```python
from build123d import *

# Parameters (mm, degrees)
SKETCH058_W     = 445
SKETCH058_H     = 232
PAD022_DEPTH    = 3
SKETCH059_R     = 9.5
POCKET036_DEPTH = 5
FILLET007_R     = 2
SKETCH060_R     = 7
POCKET037_DEPTH = 10.001
SKETCH079_W     = 462.91922
SKETCH079_H     = 530.257522
POCKET051_DEPTH = 5


with BuildPart() as part:
    # Sketch058 → Pad022 (new body)
    with BuildSketch(Plane.XY):
        Rectangle(SKETCH058_W, SKETCH058_H)
    extrude(amount=PAD022_DEPTH)

    # Sketch059 (on Face6 of Pad022) → Pocket036 (cut)
    with BuildSketch(Plane.XY.offset(3)):
        with Locations((-171, 55)):
            Circle(SKETCH059_R)
        with Locations((-171, 33)):
            Circle(SKETCH059_R)
        with Locations((-171, 11)):
            Circle(SKETCH059_R)
        with Locations((-171, -11)):
            Circle(SKETCH059_R)
        with Locations((-171, -33)):
            Circle(SKETCH059_R)
        with Locations((-171, -55)):
            Circle(SKETCH059_R)
        with Locations((-152, 44)):
            Circle(SKETCH059_R)
        with Locations((-152, 22)):
            Circle(SKETCH059_R)
        with Locations((-152, 0)):
            Circle(SKETCH059_R)
        with Locations((-152, -22)):
            Circle(SKETCH059_R)
        with Locations((-152, -44)):
            Circle(SKETCH059_R)
        with Locations((-133, 55)):
            Circle(SKETCH059_R)
        with Locations((-133, 33)):
            Circle(SKETCH059_R)
        with Locations((-133, 11)):
            Circle(SKETCH059_R)
        with Locations((-133, -11)):
            Circle(SKETCH059_R)
        with Locations((-133, -33)):
            Circle(SKETCH059_R)
        with Locations((-133, -55)):
            Circle(SKETCH059_R)
        with Locations((-114, 44)):
            Circle(SKETCH059_R)
        with Locations((-114, 22)):
            Circle(SKETCH059_R)
        with Locations((-114, 0)):
            Circle(SKETCH059_R)
        with Locations((-114, -22)):
            Circle(SKETCH059_R)
        with Locations((-114, -44)):
            Circle(SKETCH059_R)
        with Locations((-95, 55)):
            Circle(SKETCH059_R)
        with Locations((-95, 33)):
            Circle(SKETCH059_R)
        with Locations((-95, 11)):
            Circle(SKETCH059_R)
        with Locations((-95, -11)):
            Circle(SKETCH059_R)
        with Locations((-95, -33)):
            Circle(SKETCH059_R)
        with Locations((-95, -55)):
            Circle(SKETCH059_R)
        with Locations((-76, -44)):
            Circle(SKETCH059_R)
        with Locations((-76, -22)):
            Circle(SKETCH059_R)
        with Locations((-76, 0)):
            Circle(SKETCH059_R)
        with Locations((-76, 22)):
            Circle(SKETCH059_R)
        with Locations((-76, 44)):
            Circle(SKETCH059_R)
        with Locations((-57, 55)):
            Circle(SKETCH059_R)
        with Locations((-57, 33)):
            Circle(SKETCH059_R)
        with Locations((-57, 11)):
            Circle(SKETCH059_R)
        with Locations((-57, -11)):
            Circle(SKETCH059_R)
        with Locations((-57, -33)):
            Circle(SKETCH059_R)
        with Locations((-38, 44)):
            Circle(SKETCH059_R)
        with Locations((-38, 22)):
            Circle(SKETCH059_R)
        with Locations((-38, 0)):
            Circle(SKETCH059_R)
        with Locations((-38, -22)):
            Circle(SKETCH059_R)
        with Locations((-38, -44)):
            Circle(SKETCH059_R)
        with Locations((-57, -55)):
            Circle(SKETCH059_R)
        with Locations((-19, 55)):
            Circle(SKETCH059_R)
        with Locations((-19, 33)):
            Circle(SKETCH059_R)
        with Locations((-19, 11)):
            Circle(SKETCH059_R)
        with Locations((-19, -11)):
            Circle(SKETCH059_R)
        with Locations((-19, -33)):
            Circle(SKETCH059_R)
        with Locations((-19, -55)):
            Circle(SKETCH059_R)
        with Locations((0, -44)):
            Circle(SKETCH059_R)
        with Locations((0, -22)):
            Circle(SKETCH059_R)
        Circle(SKETCH059_R)
        with Locations((0, 22)):
            Circle(SKETCH059_R)
        with Locations((0, 44)):
            Circle(SKETCH059_R)
        with Locations((19, 55)):
            Circle(SKETCH059_R)
        with Locations((19, 33)):
            Circle(SKETCH059_R)
        with Locations((19, 11)):
            Circle(SKETCH059_R)
        with Locations((19, -11)):
            Circle(SKETCH059_R)
        with Locations((19, -33)):
            Circle(SKETCH059_R)
        with Locations((19, -55)):
            Circle(SKETCH059_R)
        with Locations((38, -44)):
            Circle(SKETCH059_R)
        with Locations((38, -22)):
            Circle(SKETCH059_R)
        with Locations((38, 0)):
            Circle(SKETCH059_R)
        with Locations((38, 22)):
            Circle(SKETCH059_R)
        with Locations((38, 44)):
            Circle(SKETCH059_R)
        with Locations((57, 55)):
            Circle(SKETCH059_R)
        with Locations((57, 33)):
            Circle(SKETCH059_R)
        with Locations((57, 11)):
            Circle(SKETCH059_R)
        with Locations((57, -11)):
            Circle(SKETCH059_R)
        with Locations((76, 0)):
            Circle(SKETCH059_R)
        with Locations((76, 22)):
            Circle(SKETCH059_R)
        with Locations((76, 44)):
            Circle(SKETCH059_R)
        with Locations((57, -33)):
            Circle(SKETCH059_R)
        with Locations((57, -55)):
            Circle(SKETCH059_R)
        with Locations((76, -44)):
            Circle(SKETCH059_R)
        with Locations((76, -22)):
            Circle(SKETCH059_R)
        with Locations((95, 55)):
            Circle(SKETCH059_R)
        with Locations((95, 33)):
            Circle(SKETCH059_R)
        with Locations((95, 11)):
            Circle(SKETCH059_R)
        with Locations((95, -11)):
            Circle(SKETCH059_R)
        with Locations((95, -33)):
            Circle(SKETCH059_R)
        with Locations((95, -55)):
            Circle(SKETCH059_R)
        with Locations((114, 44)):
            Circle(SKETCH059_R)
        with Locations((114, 22)):
            Circle(SKETCH059_R)
        with Locations((114, 0)):
            Circle(SKETCH059_R)
        with Locations((114, -22)):
            Circle(SKETCH059_R)
        with Locations((114, -44)):
            Circle(SKETCH059_R)
        with Locations((133, 55)):
            Circle(SKETCH059_R)
        with Locations((133, 33)):
            Circle(SKETCH059_R)
        with Locations((133, 11)):
            Circle(SKETCH059_R)
        with Locations((133, -11)):
            Circle(SKETCH059_R)
        with Locations((133, -33)):
            Circle(SKETCH059_R)
        with Locations((133, -55)):
            Circle(SKETCH059_R)
        with Locations((152, 44)):
            Circle(SKETCH059_R)
        with Locations((152, 22)):
            Circle(SKETCH059_R)
        with Locations((152, 0)):
            Circle(SKETCH059_R)
        with Locations((152, -22)):
            Circle(SKETCH059_R)
        with Locations((152, -44)):
            Circle(SKETCH059_R)
        with Locations((171, 55)):
            Circle(SKETCH059_R)
        with Locations((171, 33)):
            Circle(SKETCH059_R)
        with Locations((171, 11)):
            Circle(SKETCH059_R)
        with Locations((171, -11)):
            Circle(SKETCH059_R)
        with Locations((171, -33)):
            Circle(SKETCH059_R)
        with Locations((171, -55)):
            Circle(SKETCH059_R)
    extrude(amount=-POCKET036_DEPTH, mode=Mode.SUBTRACT)

    # Fillet007
    fillet007_edges = [part.edges().sort_by_distance(p)[0] for p in [
        (-222.5, -116, 1.5),
        (222.5, -116, 1.5),
        (222.5, 116, 1.5),
        (-222.5, 116, 1.5),
    ]]
    fillet(fillet007_edges, radius=FILLET007_R)

    # Sketch060 → Pocket037 (cut, through all)
    with BuildSketch(Plane.XY.offset(10)):
        with Locations((197.939534, 0)):
            Circle(SKETCH060_R)
    extrude(amount=-POCKET037_DEPTH, mode=Mode.SUBTRACT)

    # Sketch079 (on Face5 of Pocket037) → Pocket051 (cut)
    with BuildSketch(Plane.XY.offset(3)):
        with Locations((-171.45961, -16.154991)):
            Rectangle(SKETCH079_W, SKETCH079_H)
    extrude(amount=-POCKET051_DEPTH, mode=Mode.SUBTRACT)


solid = part.part
```
Verification items for the finished model (mm, model axes). Give positions to 0.01 mm unless a question says otherwise; leave off trailing zeros. Order: outer loops, then holes, each group sorted by start corner. A loop starts at its lowest first (then second) coordinate and runs counter-clockwise, first axis right, second up. Notation, with made-up numbers: M 10,33 L 19,33 A8 ccw 19,37 Z; hole C -33,52.5 d6. An arc over 180 degrees is marked long. Answer in a Markdown table with one row per item. Add a question column.
Item 1: Mould release check, pull along Y, two halves, no side actions. Record for faces 1 (the cylindrical face through (123.51, -10.58, 1.52)), 2 (the flat face through (140, 2, 0)): released by +Y, released by -Y, zero draft, split by the parting line, or undercut.
Item 2: Section check C-C, the plane y = -28. Enter the section's corners in (x, z).
Item 3: Gauge pin test, flat end, axial feed: pin 1 (11.5 mm diameter, centred on x = 95, y = 33, fed in from -Z). Record the tip position at first contact, or that the pin passes through.
Item 4: Section check D-D, the plane z = 1.3. State how many separate pieces and enclosed holes the cut face has, and give its area (3 significant figures).
Item 5: Section check A-A, the plane x = 152. Enter the section's corners in (y, z), and give its area (3 significant figures).
Item 6: Section check B-B, the plane x = 174. Enter the section's corners in (y, z), and give its area (4 significant figures).
Item 7: Scan lines: probe 1 along Y at (x, z) = (76, 0.8); probe 2 along X at (y, z) = (-57.5, 2.7); probe 3 along Y at (x, z) = (72, 1.5). Record each from-to range of solid material in increasing order. Write a range as from..to.
Filled sheet:
| question | item | result |
|---|---|---|
| 1 | face 1 | undercut |
| 1 | face 2 | zero draft |
| 2 | outline | M 65.08,0 L 68.63,0 L 68.63,3 L 65.08,3 Z; M 83.37,0 L 86.92,0 L 86.92,3 L 83.37,3 Z; M 103.08,0 L 106.63,0 L 106.63,3 L 103.08,3 Z; M 121.37,0 L 124.92,0 L 124.92,3 L 121.37,3 Z; M 141.08,0 L 144.63,0 L 144.63,3 L 141.08,3 Z; M 159.37,0 L 162.92,0 L 162.92,3 L 159.37,3 Z; M 179.08,0 L 222.5,0 L 222.5,3 L 179.08,3 Z |
| 3 | pin 1 | passes through |
| 4 | separate pieces | 1 |
| 4 | enclosed holes | 34 |
| 4 | area | 27,700 mm^2 |
| 5 | outline | M -116,0 L -53.5,0 L -53.5,3 L -116,3 Z; M -34.5,0 L -31.5,0 L -31.5,3 L -34.5,3 Z; M -12.5,0 L -9.5,0 L -9.5,3 L -12.5,3 Z; M 9.5,0 L 12.5,0 L 12.5,3 L 9.5,3 Z; M 31.5,0 L 34.5,0 L 34.5,3 L 31.5,3 Z; M 53.5,0 L 116,0 L 116,3 L 53.5,3 Z |
| 5 | area | 411 mm^2 |
| 6 | outline | M -116,0 L -64.01,0 L -64.01,3 L -116,3 Z; M -45.99,0 L -42.01,0 L -42.01,3 L -45.99,3 Z; M -23.99,0 L -20.01,0 L -20.01,3 L -23.99,3 Z; M -1.99,0 L 1.99,0 L 1.99,3 L -1.99,3 Z; M 20.01,0 L 23.99,0 L 23.99,3 L 20.01,3 Z; M 42.01,0 L 45.99,0 L 45.99,3 L 42.01,3 Z; M 64.01,0 L 116,0 L 116,3 L 64.01,3 Z |
| 6 | area | 371.5 mm^2 |
| 7 | probe 1 | y = -116..-53.5, -34.5..-31.5, -12.5..-9.5, 9.5..12.5, 31.5..34.5, 53.5..116 |
| 7 | probe 2 | x = 66.17..85.83, 104.17..123.83, 142.17..161.83, 180.17..222.5 |
| 7 | probe 3 | y = -116..-52.62, -35.38..-30.62, -13.38..-8.62, 8.62..13.38, 30.62..35.38, 52.62..116 |
